Read the model definition and answer for the solid it produces. Units are mm, in the model's axes. Coordinates: 2 decimals unless noted, no trailing zeros. Order: outer loops, then holes, each group sorted by start corner. A loop starts at its lowest first (then second) coordinate and runs counter-clockwise, first axis right, second up. Notation, with made-up numbers: M -18,13.25 L 20,13.25 A16 cw 20,29.25 Z; hole C 64,5 d8. An arc over 180 degrees is marked long. Put each result on its own line as item: value.
from build123d import *

# Parameters (mm, degrees)
SKETCH1_W                         = 25.4
SKETCH1_H                         = 88.9
BOSS_EXTRUDE1_DEPTH               = 6.35
F_1_4_20_TAPPED_HOLE1_D           = 5.1054
F_1_4_20_TAPPED_HOLE1_CSINK_D     = 7.62
F_1_4_20_TAPPED_HOLE1_CSINK_ANGLE = 90
F_3_8_16_TAPPED_HOLE1_D           = 7.9375
F_3_8_16_TAPPED_HOLE1_CSINK_D     = 10.795
F_3_8_16_TAPPED_HOLE1_CSINK_ANGLE = 90


with BuildPart() as part:
    # Sketch1 → Boss-Extrude1 (new body)
    with BuildSketch(Plane(origin=(0, 0, 0), x_dir=(1, 0, 0), z_dir=(0, 1, 0))):
        with Locations((-12.7, 44.45)):
            Rectangle(SKETCH1_W, SKETCH1_H)
    extrude(amount=BOSS_EXTRUDE1_DEPTH)

    # 1/4-20 Tapped Hole1 (through all)
    with Locations(Plane(origin=(0, 6.35, 0), x_dir=(1, 0, 0), z_dir=(0, 1, 0))):
        with Locations((-13.284419072, 15.875), (-13.284419072, 44.45)):
            CounterSinkHole(F_1_4_20_TAPPED_HOLE1_D / 2, F_1_4_20_TAPPED_HOLE1_CSINK_D / 2, counter_sink_angle=F_1_4_20_TAPPED_HOLE1_CSINK_ANGLE)

    # 3/8-16 Tapped Hole1 (through all)
    with Locations(Plane(origin=(0, 6.35, 0), x_dir=(1, 0, 0), z_dir=(0, 1, 0))):
        with Locations((-13.284419072, 73.025)):
            CounterSinkHole(F_3_8_16_TAPPED_HOLE1_D / 2, F_3_8_16_TAPPED_HOLE1_CSINK_D / 2, counter_sink_angle=F_3_8_16_TAPPED_HOLE1_CSINK_ANGLE)


solid = part.part
Q1. Find section B-B on y = 2.75. Give the number of separate pieces and of enclosed holes in the cut face, plus the area to 3 significant figures.
Answers below:
separate pieces: 1
enclosed holes: 3
area: 2,170 mm^2
Q2. Given pin 1 (5 mm diameter, centred on x = -13.28, z = -73.03, fed in from -Y), flat-ended and moving along its own axis, determine where the tip first touches the part or whether it passes through.
Answers below:
pin 1: passes through
Q3. For a pull along X with two mould halves and no side action, classify faces 1 (the face through (-13, 3, -88.9)), 2 (the face through (-25.4, 3, -44)), 3 (the face through (-12.42, 2.43, -69.15)) as +X half, -X half, draft (parallel to the pull), parting line (faces both ways), or undercut.
Answers below:
face 1: draft
face 2: -X half
face 3: undercut
Q4. Find section A-A on z = -44.45. Write down the section's boundary in (x, y), plus the area to 3 significant figures.
Answers below:
outline: M -25.4,0 L -15.84,0 L -15.84,5.09 L -17.09,6.35 L -25.4,6.35 Z; M -10.73,0 L 0,0 L 0,6.35 L -9.47,6.35 L -10.73,5.09 Z
area: 127 mm^2
Q5. Consider line 1 along Z through (x, y) = (-11.5, 1.75); line 2 along Z through (x, y) = (-14.5, 4.5); line 3 along X through (y, z) = (2.25, -44). Determine where each line is inside the solid, lowest interval first.
Answers below:
line 1: z = -88.9 to -76.57, -69.48 to -46.28, -42.62 to -17.7, -14.05 to 0
line 2: z = -88.9 to -76.8, -69.25 to -46.69, -42.21 to -18.12, -13.63 to 0
line 3: x = -25.4 to -15.8, -10.77 to 0
